from build123d import *

# Parameters (mm, degrees)
SKETCH2_W           = 76.2
SKETCH2_H           = 101.6
BOSS_EXTRUDE1_DEPTH = 4.7752
SKETCH3_W           = 25.4
SKETCH3_H           = 4.7752
SKETCH3_W_2         = 38.1
CUT_EXTRUDE1_DEPTH  = 6.35
SKETCH4_W           = 4.7752
SKETCH4_H           = 26.9748
SKETCH4_H_2         = 12.7
SKETCH4_H_3         = 6.35
SKETCH4_H_4         = 19.05
CUT_EXTRUDE2_DEPTH  = 6.35
SKETCH6_W           = 12.7
SKETCH6_H           = 4.775408317
CUT_EXTRUDE4_DEPTH  = 4.7752


with BuildPart() as part:
    # Sketch2 → Boss-Extrude1 (new body)
    with BuildSketch(Plane(origin=(0, 0, 0), x_dir=(0, 0, -1), z_dir=(1, 0, 0))):
        with Locations((38.1, 50.8)):
            Rectangle(SKETCH2_W, SKETCH2_H)
    extrude(amount=BOSS_EXTRUDE1_DEPTH)

    # Sketch3 → Cut-Extrude1 (cut)
    with BuildSketch(Plane(origin=(4.7752, 0, 0), x_dir=(0, 0, -1), z_dir=(1, 0, 0))):
        with Locations((12.7, 2.3876)):
            Rectangle(SKETCH3_W, SKETCH3_H)
        with Locations((57.15, 2.3876)):
            Rectangle(SKETCH3_W_2, SKETCH3_H)
    extrude(amount=-CUT_EXTRUDE1_DEPTH, mode=Mode.SUBTRACT)

    # Sketch4 → Cut-Extrude2 (cut)
    with BuildSketch(Plane(origin=(4.7752, 0, 0), x_dir=(0, 0, -1), z_dir=(1, 0, 0))):
        with Locations((2.3876, 88.1126)):
            Rectangle(SKETCH4_W, SKETCH4_H)
        with Locations((73.8124, 95.25)):
            Rectangle(SKETCH4_W, SKETCH4_H_2)
        with Locations((73.8124, 69.85)):
            Rectangle(SKETCH4_W, SKETCH4_H_2)
        with Locations((2.3876, 7.9502)):
            Rectangle(SKETCH4_W, SKETCH4_H_3)
        with Locations((73.8124, 14.3002)):
            Rectangle(SKETCH4_W, SKETCH4_H_4)
        with Locations((73.8124, 44.45)):
            Rectangle(SKETCH4_W, SKETCH4_H_2)
        with Locations((2.3876, 55.5752)):
            Rectangle(SKETCH4_W, SKETCH4_H_2)
        with Locations((2.3876, 30.1752)):
            Rectangle(SKETCH4_W, SKETCH4_H_2)
    extrude(amount=-CUT_EXTRUDE2_DEPTH, mode=Mode.SUBTRACT)

    # Sketch6 → Cut-Extrude4 (cut)
    with BuildSketch(Plane(origin=(4.7752, 0, 0), x_dir=(0, 0, -1), z_dir=(1, 0, 0))):
        with Locations((27.7876, 99.212295842)):
            Rectangle(SKETCH6_W, SKETCH6_H)
        with Locations((15.0876, 99.212295842)):
            Rectangle(SKETCH6_W, SKETCH6_H)
        with Locations((48.4124, 99.212295842)):
            Rectangle(SKETCH6_W, SKETCH6_H)
        with Locations((61.1124, 99.212295842)):
            Rectangle(SKETCH6_W, SKETCH6_H)
    extrude(amount=-CUT_EXTRUDE4_DEPTH, mode=Mode.SUBTRACT)


solid = part.part
Verification items for the finished model (mm, model axes). A direction names the side the tool comes from. Round coordinates to 2 decimals unless told otherwise and drop trailing zeros. Order: outer loops, then holes, each group sorted by start corner. A loop starts at its lowest first (then second) coordinate and runs counter-clockwise, first axis right, second up.
1. Release check for a two-part mould opening along Y. For faces 1 (the flat face through (2, 70, -71.425)), 2 (the flat face through (2, 96.825, -55)), 3 (the flat face through (2, 4.775, -15)) record: +Y half, -Y half, draft (parallel to the pull), parting line (faces both ways), or undercut.
Final values:
face 1: undercut
face 2: +Y half
face 3: -Y half
2. Section check A-A on y = 17. Record the cut outline in (x, z), then the cut area to 3 significant figures.
Final values:
outline: (0, -71.42) - (4.78, -71.42) - (4.78, 0) - (0, 0) - close
area: 341 mm2
3. Section check B-B on z = -30.5. Record the cut outline in (x, y).
Final values:
outline: (0, 0) - (4.78, 0) - (4.78, 96.82) - (0, 96.82) - close
4. Access from +Z, -Z, +X, -X, +Y, -Y to the whole of each face (thin tool, end or side, straight path). Record for faces 4 (the flat face through (2, 14, -71.425)), 5 (the flat face through (2, 23.825, -2)), 6 (the flat face through (2, 74.625, -2)), 7 (the flat face through (2, 44, -71.425)), 8 (the flat face through (2, 2, -25.4)).
Final values:
face 4: -Z, +X, -X, -Y
face 5: +Z, +X, -X
face 6: +Z, +X, -X, +Y
face 7: -Z, +X, -X
face 8: +Z, +X, -X, -Y
5. Thickness scan on L1, parallel to Y at x = 1.45, z = -63; L2, parallel to Z at x = 2.2, y = 91.5; L3, parallel to Z at x = 1.45, y = 29. Record the ranges inside material, lowest first.
Final values:
L1: y = 4.78 to 96.82
L2: z = -71.42 to -4.78
L3: z = -76.2 to -4.78
6. Go/stop test with flat-tipped pins: P1, Ø1, axis at x = 4, y = 65, coming from the -Z side; P2, Ø2.5, axis at x = 3, z = -2, coming from the -Y side; P3, Ø2.5, axis at x = 2.5, z = -2, coming from the +Y side. Record where each tip stops, or that it passes through.
Final values:
P1: stops at z = -71.42
P2: stops at y = 11.13
P3: stops at y = 74.63
